from build123d import *

# Parameters (mm, degrees)
SKETCH4_R           = 150
SKETCH4_R_2         = 65
BOSS_EXTRUDE3_DEPTH = 40
SKETCH5_R           = 50
CUT_EXTRUDE1_DEPTH  = 11
SKETCH6_R           = 65
CUT_EXTRUDE2_DEPTH  = 121


with BuildPart() as part:
    # Sketch1 → Revolve2 (revolve)
    with BuildSketch(Plane.XY):
        with BuildLine():
            Line((-200, 10), (-200, 0))
            Line((-200, 0), (200, 0))
            Line((200, 0), (200, 10))
            Line((200, 10), (165, 10))
            Line((165, 10), (165, 50))
            ThreePointArc((165, 50), (156.213203436, 71.213203436), (135, 80))
            Line((135, 80), (50, 80))
            Line((50, 80), (50, 95))
            Line((50, 95), (-50, 95))
            Line((-50, 95), (-50, 80))
            Line((-50, 80), (-135, 80))
            ThreePointArc((-135, 80), (-156.213203436, 71.213203436), (-165, 50))
            Line((-165, 50), (-165, 10))
            Line((-165, 10), (-200, 10))
        make_face()
    revolve(axis=Axis((-200, -16.726974685, 0), (0, 1, 0)))

    # Sketch4 → Boss-Extrude3 (add)
    with BuildSketch(Plane(origin=(0, 80, 0), x_dir=(1, 0, 0), z_dir=(0, 1, 0))):
        with Locations((-200, 0)):
            Circle(SKETCH4_R)
        with Locations((-200, 0)):
            Circle(SKETCH4_R_2, mode=Mode.SUBTRACT)
    extrude(amount=BOSS_EXTRUDE3_DEPTH)

    # Sketch5 → Cut-Extrude1 (cut, through all)
    with BuildSketch(Plane(origin=(0, 10, 0), x_dir=(1, 0, 0), z_dir=(0, 1, 0))):
        with Locations((-200, 0)):
            Circle(SKETCH5_R)
    extrude(amount=-CUT_EXTRUDE1_DEPTH, mode=Mode.SUBTRACT)

    # Sketch6 → Cut-Extrude2 (cut, through all)
    with BuildSketch(Plane(origin=(0, 120, 0), x_dir=(1, 0, 0), z_dir=(0, 1, 0))):
        with Locations((-200, 0)):
            Circle(SKETCH6_R)
    extrude(amount=-CUT_EXTRUDE2_DEPTH, mode=Mode.SUBTRACT)


solid = part.part
Model file for the job. Use its own axes, mm. A direction names the side the tool comes from. Round coordinates to 2 decimals unless told otherwise and drop trailing zeros. Loops run counter-clockwise (first coordinate to the right, second up) from the corner with the lowest first, then second, coordinate; pieces in that order, holes last.
1. Band-saw the part on C-C, the plane y = 23. List the corners of the cut face in (x, z).
Check values:
outline: circle Ø730 at (-200, 0); hole circle Ø130 at (-200, 0)
2. Band-saw the part on B-B, the plane x = -200. List the corners of the cut face in (y, z).
Check values:
outline: (0, -400) - (10, -400) - (10, -365) - (50, -365) arc R30 ccw to (80, -335) - (80, -250) - (95, -250) - (95, -150) - (120, -150) - (120, -65) - (0, -65) - close; (0, 65) - (120, 65) - (120, 150) - (95, 150) - (95, 250) - (80, 250) - (80, 335) arc R30 ccw to (50, 365) - (10, 365) - (10, 400) - (0, 400) - close
3. Tool access for faces 1 (the cylindrical face through (-449.76, 87.6, -10.99)), 2 (the flat face through (-135, 120, 31)): list every direction of +Z, -Z, +X, -X, +Y, -Y with a clear straight run to the whole face (end or side of a thin tool).
Check values:
face 1: +Y
face 2: +Z, -Z, +X, -X, +Y
4. Drop flat-ended pins along their axis: P1, Ø8, axis at x = -400.5, y = 34, coming from the -Z side; P2, Ø6, axis at y = 21, z = 55.5, coming from the -X side; P3, Ø12, axis at x = -271, y = 74.5, coming from the -Z side. Give the stop position or say it passes through.
Check values:
P1: stops at z = -307.59
P2: stops at x = -561.2
P3: stops at z = -351.66
5. Wall check: probe 1 along Z at (x, y) = (-200, 21); probe 2 along X at (y, z) = (110, 0); probe 3 along Y at (x, z) = (-16.5, -282.5). Give the ranges that are in metal, low to high.
Check values:
probe 1: z = -365 to -65, 65 to 365
probe 2: x = -350 to -265, -135 to -50
probe 3: y = 0 to 79.94
6. Band-saw the part on A-A, the plane z = 0. List the corners of the cut face in (x, y).
Check values:
outline: (-600, 0) - (-265, 0) - (-265, 120) - (-350, 120) - (-350, 95) - (-450, 95) - (-450, 80) - (-535, 80) arc R30 ccw to (-565, 50) - (-565, 10) - (-600, 10) - close; (-135, 0) - (200, 0) - (200, 10) - (165, 10) - (165, 50) arc R30 ccw to (135, 80) - (50, 80) - (50, 95) - (-50, 95) - (-50, 120) - (-135, 120) - close
